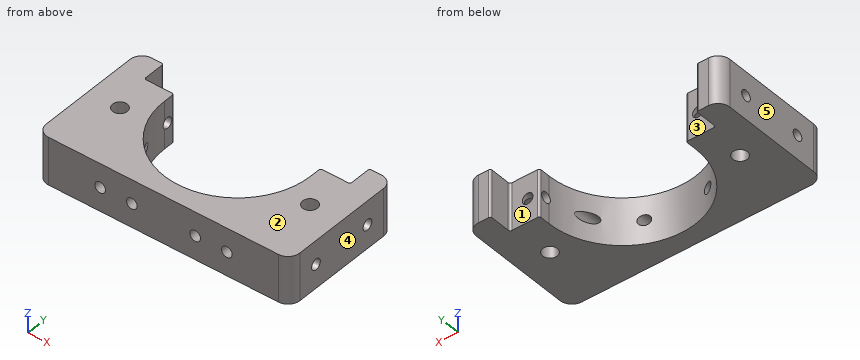
from build123d import *

# Parameters (mm, degrees)
SKETCH1_W                  = 64
SKETCH1_H                  = 32
BOSS_EXTRUDE1_DEPTH        = 12
CUT_EXTRUDE1_DEPTH         = 43.941821107
SKETCH3_W                  = 7.5
SKETCH3_H                  = 6
CUT_EXTRUDE2_DEPTH         = 43.941821107
M2_5_CLEARANCE_HOLE1_D     = 2.7051
M2_5_CLEARANCE_HOLE1_DEPTH = 32
M2_5_CLEARANCE_HOLE2_D     = 2.7051
M2_5_CLEARANCE_HOLE2_DEPTH = 32
F_3_7_3_7_DIAMETER_HOLE1_D = 3.7
M2_5_CLEARANCE_HOLE3_D     = 2.7051
M2_5_CLEARANCE_HOLE3_DEPTH = 12
M2_5_CLEARANCE_HOLE3_TIP   = 0.560244554
F_3_7_3_7_DIAMETER_HOLE2_D = 3.7
M2_5_CLEARANCE_HOLE4_D     = 2.7051
M2_5_CLEARANCE_HOLE4_DEPTH = 74.5
M2_5_CLEARANCE_HOLE5_D     = 2.7051
M2_5_CLEARANCE_HOLE5_DEPTH = 10.5
M2_5_CLEARANCE_HOLE5_TIP   = 0.560244554
M2_5_CLEARANCE_HOLE6_D     = 2.7051
M2_5_CLEARANCE_HOLE6_DEPTH = 10.5
M2_5_CLEARANCE_HOLE6_TIP   = 0.560244554
FILLET1_R                  = 0.5
FILLET2_R                  = 3


with BuildPart() as part:
    # Sketch1 → Boss-Extrude1 (new body)
    with BuildSketch(Plane(origin=(0, 0, -6), x_dir=(-1, 0, 0), z_dir=(0, 0, -1))):
        with Locations((0, -10)):
            Rectangle(SKETCH1_W, SKETCH1_H)
    extrude(amount=-BOSS_EXTRUDE1_DEPTH)

    # Sketch2 → Cut-Extrude1 (cut, through all)
    with BuildSketch(Plane.XY.offset(6)):
        with BuildLine():
            Line((-26, 6), (-26, 0))
            Line((-26, 0), (-18.5, 0))
            Line((-18.5, 0), (-18.5, -3))
            ThreePointArc((-18.5, -3), (0, -21.5), (18.5, -3))
            Line((18.5, -3), (18.5, 6))
            Line((18.5, 6), (-26, 6))
        make_face()
    extrude(amount=-CUT_EXTRUDE1_DEPTH, mode=Mode.SUBTRACT)

    # Sketch3 → Cut-Extrude2 (cut, through all)
    with BuildSketch(Plane.XY.offset(6)):
        with Locations((22.25, 3)):
            Rectangle(SKETCH3_W, SKETCH3_H)
    extrude(amount=-CUT_EXTRUDE2_DEPTH, mode=Mode.SUBTRACT)

    # M2.5 Clearance Hole1
    with Locations(Plane(origin=(0, -26, 0), x_dir=(-1, 0, 0), z_dir=(0, -1, 0))):
        with Locations((8, 0), (-8, 0)):
            Hole(M2_5_CLEARANCE_HOLE1_D / 2, depth=M2_5_CLEARANCE_HOLE1_DEPTH)

    # M2.5 Clearance Hole2
    with Locations(Plane(origin=(0, -26, 0), x_dir=(-1, 0, 0), z_dir=(0, -1, 0))):
        with Locations((16, 0), (-16, 0)):
            Hole(M2_5_CLEARANCE_HOLE2_D / 2, depth=M2_5_CLEARANCE_HOLE2_DEPTH)

    # Ø3.7 (3.7) Diameter Hole1 (through all)
    with Locations(Plane(origin=(0, 0, -6), x_dir=(-1, 0, 0), z_dir=(0, 0, -1))):
        with Locations((24, -10)):
            Hole(F_3_7_3_7_DIAMETER_HOLE1_D / 2)

    # M2.5 Clearance Hole3
    with Locations(Plane(origin=(0, 0, 0), x_dir=(1, 0, 0), z_dir=(0, 1, 0))):
        with Locations((21.5, 0), (-21.5, 0)):
            Hole(M2_5_CLEARANCE_HOLE3_D / 2, depth=M2_5_CLEARANCE_HOLE3_DEPTH)
            with Locations((0, 0, -(M2_5_CLEARANCE_HOLE3_DEPTH + M2_5_CLEARANCE_HOLE3_TIP / 2))):  # 135° drill point
                Cone(0, M2_5_CLEARANCE_HOLE3_D / 2, M2_5_CLEARANCE_HOLE3_TIP, mode=Mode.SUBTRACT)

    # Ø3.7 (3.7) Diameter Hole2 (through all)
    with Locations(Plane.XY.offset(6)):
        with Locations((24, -10)):
            Hole(F_3_7_3_7_DIAMETER_HOLE2_D / 2)

    # M2.5 Clearance Hole4
    with Locations(Plane(origin=(32, 0, 0), x_dir=(0, 0, -1), z_dir=(1, 0, 0))):
        with Locations((0, -2)):
            Hole(M2_5_CLEARANCE_HOLE4_D / 2, depth=M2_5_CLEARANCE_HOLE4_DEPTH)

    # M2.5 Clearance Hole5
    with Locations(Plane(origin=(32, 0, 0), x_dir=(0, 0, -1), z_dir=(1, 0, 0))):
        with Locations((0, -18)):
            Hole(M2_5_CLEARANCE_HOLE5_D / 2, depth=M2_5_CLEARANCE_HOLE5_DEPTH)
            with Locations((0, 0, -(M2_5_CLEARANCE_HOLE5_DEPTH + M2_5_CLEARANCE_HOLE5_TIP / 2))):  # 135° drill point
                Cone(0, M2_5_CLEARANCE_HOLE5_D / 2, M2_5_CLEARANCE_HOLE5_TIP, mode=Mode.SUBTRACT)

    # M2.5 Clearance Hole6
    with Locations(Plane.ZY.offset(32)):
        with Locations((0, -18)):
            Hole(M2_5_CLEARANCE_HOLE6_D / 2, depth=M2_5_CLEARANCE_HOLE6_DEPTH)
            with Locations((0, 0, -(M2_5_CLEARANCE_HOLE6_DEPTH + M2_5_CLEARANCE_HOLE6_TIP / 2))):  # 135° drill point
                Cone(0, M2_5_CLEARANCE_HOLE6_D / 2, M2_5_CLEARANCE_HOLE6_TIP, mode=Mode.SUBTRACT)

    # Fillet1
    fillet1_edges = [part.edges().sort_by_distance(p)[0] for p in [
        (-26, 6, 0),
        (-18.5, 0, 0),
        (-26, 0, 0),
        (18.5, 0, 0),
        (26, 6, 0),
        (26, 0, 0),
    ]]
    fillet(fillet1_edges, radius=FILLET1_R)

    # Fillet2
    fillet2_edges = [part.edges().sort_by_distance(p)[0] for p in [
        (32, -26, 0),
        (32, 6, 0),
        (-32, 6, 0),
        (-32, -26, 0),
    ]]
    fillet(fillet2_edges, radius=FILLET2_R)


solid = part.part
Read the model definition and answer for the solid it produces. Units are mm, in the model's axes. Face numbers are marked on the shaded views. A direction names the side the tool comes from. Coordinates: 2 decimals unless noted, no trailing zeros. Loops run counter-clockwise (first coordinate to the right, second up) from the corner with the lowest first, then second, coordinate; pieces in that order, holes last. Notation, with made-up numbers: (47, 3.5) - (98, 3.5) arc R16 cw to (98, 32.5) - close; hole circle Ø7 at (60.25, 23.25). An arc over 180 degrees is marked (long way). Answer in a Markdown table with one row per item.
Q1. The mould has two halves that part along X. Classify the marked faces 3, 4 and 5: pulls with the +X half, pulls with the -X half, needs draft (parallel to the pull), parting line crosses it, or undercut.
Here are the results:
| item | result |
|---|---|
| face 3 | undercut |
| face 4 | pulls with the +X half |
| face 5 | pulls with the -X half |
Q2. For the marked faces 1 and 2, determine the directions among +Z, -Z, +X, -X, +Y, -Y from which every point of the face is accessible in a straight line to the end or side of a thin tool.
Here are the results:
| item | result |
|---|---|
| face 1 | +Z, -Z, +Y |
| face 2 | +Z, +X, -X, +Y, -Y |
Q3. Find section B-B on z = -4.5. Write down the section's boundary in (x, y), plus the area to 3 significant figures.
Here are the results:
| item | result |
|---|---|
| outline | (-32, -23) arc R3 ccw to (-29, -26) - (29, -26) arc R3 ccw to (32, -23) - (32, 3) arc R3 ccw to (29, 6) - (26.5, 6) arc R0.5 ccw to (26, 5.5) - (26, 0.5) arc R0.5 cw to (25.5, 0) - (19, 0) arc R0.5 ccw to (18.5, -0.5) - (18.5, -3) arc R18.5 cw to (-18.5, -3) - (-18.5, -0.5) arc R0.5 ccw to (-19, 0) - (-25.5, 0) arc R0.5 cw to (-26, 0.5) - (-26, 5.5) arc R0.5 ccw to (-26.5, 6) - (-29, 6) arc R3 ccw to (-32, 3) - close; hole circle Ø3.7 at (-24, -10); hole circle Ø3.7 at (24, -10) |
| area | 1,060 mm^2 |
Q4. Find section C-C on y = -15. Write down the section's boundary in (x, z).
Here are the results:
| item | result |
|---|---|
| outline | (-32, -6) - (-14.08, -6) - (-14.08, 6) - (-32, 6) - close; (14.08, -6) - (32, -6) - (32, 6) - (14.08, 6) - close; hole circle Ø2.71 at (-16, 0); hole circle Ø2.71 at (16, 0) |
Q5. Given P1, Ø2, axis at y = -18, z = 0, coming from the -X side; P2, Ø3, axis at x = 22.5, z = 1, coming from the +Y side; P3, Ø2, axis at x = -21.5, z = 0, coming from the +Y side; P4, Ø1.6, axis at x = -16, z = 0, coming from the -Y side, each flat-ended and moving along its own axis, determine where each tip first touches the part or whether it passes through.
Here are the results:
| item | result |
|---|---|
| P1 | stops at x = -21.35 |
| P2 | stops at y = 0 |
| P3 | stops at y = -12.15 |
| P4 | passes through |
Q6. Find section D-D on x = -16. Write down the section's boundary in (y, z), plus the area to 3 significant figures.
Here are the results:
| item | result |
|---|---|
| outline | (-26, -6) - (-12.29, -6) - (-12.29, -1.35) - (-26, -1.35) - close; (-26, 1.35) - (-12.29, 1.35) - (-12.29, 6) - (-26, 6) - close |
| area | 127 mm^2 |
Q7. Find section A-A on x = -24. Write down the section's boundary in (y, z), plus the area to 3 significant figures.
Here are the results:
| item | result |
|---|---|
| outline | (-26, -6) - (-11.85, -6) - (-11.85, 6) - (-26, 6) - close; (-8.15, -6) - (0, -6) - (0, 6) - (-8.15, 6) - close; hole circle Ø2.71 at (-18, 0); hole circle Ø2.71 at (-2, 0) |
| area | 256 mm^2 |
Q8. Straight lines are drawn through the part: line 1 along Y through (x, z) = (-26.5, 0); line 2 along X through (y, z) = (0.5, 4.25); line 3 along Z through (x, y) = (19.55, -2). For each, find the intervals that lie inside material, in ascending order. Write a range as [from, to].
Here are the results:
| item | result |
|---|---|
| line 1 | y = [-26, -19.35], [-16.65, -3.35], [-0.65, 6] |
| line 2 | x = [-32, -26], [26, 32] |
| line 3 | z = [-6, -1.35], [1.35, 6] |
